Work out the finished part from the listing and answer in its coordinate system (mm). A direction names the side the tool comes from. Round coordinates to 2 decimals unless told otherwise and drop trailing zeros. Order: outer loops, then holes, each group sorted by start corner. A loop starts at its lowest first (then second) coordinate and runs counter-clockwise, first axis right, second up. Notation, with made-up numbers: (-14, 80.5) -> (-1, 80.5) arc R22 cw to (-1, 86.5) -> close; hole circle Ø10 at (53, 13.5). An arc over 180 degrees is marked (long way). Use a Markdown table: item, result. Add a question column.
Item 1: A cutting plane is placed at B-B, the plane y = -11.5. Determine the outline of the cut face in (x, z).
Item 2: A tool of negligible diameter and unlimited length cuts with its end or side. For faces 1 (the flat face through (6, 16, -0.15)), 2 (the cylindrical face through (-0.81, 18.34, -0.07)), 3 (the flat face through (0.996, 16.1, -6.2)), from which of +Z, -Z, +X, -X, +Y, -Y can it reach the whole face along a straight path? Write none if from no direction.
Item 3: A cutting plane is placed at A-A, the plane x = -13. Determine the outline of the cut face in (y, z).
Item 4: Find the intervals of material crossed by L1, parallel to Z at x = 1.2, y = 0; L2, parallel to Y at x = 2.5, z = 0; L3, parallel to X at y = -15, z = -4.5, in increasing order. Write a range as [from, to].
Item 5: A cutting plane is placed at C-C, the plane y = 8. Determine the outline of the cut face in (x, z).
Item 6: Flat-ended cylindrical pins translate along their axes: P1, Ø18, axis at y = 0, z = 0, coming from the +X side; P2, Ø3, axis at x = -3, y = 12.5, coming from the -Z side; P3, Ø3, axis at y = 17, z = 5.5, coming from the -X side; P4, Ø2.5, axis at y = 0, z = -22, coming from the +X side. Find the tip coordinate at first contact, or state that the pin passes through.
Item 7: For a pull along Y with two mould halves and no side action, classify faces 4 (the cylindrical face through (2.03, 0.07, 23.5)), 5 (the cylindrical face through (-7.643, 11.528, 0.14)), 6 (the cylindrical face through (1.97, 6.45, -17.26)), 7 (the flat face through (4, 0, -20)) as +Y half, -Y half, draft (parallel to the pull), parting line (faces both ways), or undercut.
from build123d import *

# Parameters (mm, degrees)
SKETCH_1_R          = 17
EXTRUDE_1_DEPTH     = 7
EXTRUDE_2_DEPTH     = 4
SKETCH_2_R          = 15
CUT_EXTRUDE_1_DEPTH = 3
CUT_EXTRUDE_2_REACH = 33.321
SKETCH_3_R          = 5.15
SKETCH_4_R          = 13
CUT_EXTRUDE_3_DEPTH = 2
CUT_EXTRUDE_4_REACH = 33.321
SKETCH_6_R          = 1.5
FILLET_1_R          = 10
FILLET_2_R          = 5
SKETCH_8_W          = 0.3
SKETCH_8_H          = 2.22932804
CUT_EXTRUDE_5_DEPTH = 3
SKETCH_9_W          = 20
SKETCH_9_H          = 2.594823192
EXTRUDE_3_DEPTH     = 8
SKETCH_10_W         = 5.99596414
SKETCH_10_H         = 20
EXTRUDE_4_DEPTH     = 8
SKETCH_11_W         = 20
SKETCH_11_H         = 6
EXTRUDE_5_DEPTH     = 10
SKETCH_12_R         = 3
CUT_EXTRUDE_6_DEPTH = 10
FILLET_3_R          = 10
EXTRUDE_6_DEPTH     = 3
FILLET_5_R          = 5
FILLET_6_R          = 5
FILLET_7_R          = 8
FILLET_9_R          = 2


with BuildPart() as part:
    # 草图1 → 凸台-拉伸1 (new body)
    with BuildSketch(Plane(origin=(0, 0, 0), x_dir=(0, 0, -1), z_dir=(1, 0, 0))):
        Circle(SKETCH_1_R)
    extrude(amount=EXTRUDE_1_DEPTH)

    # 草图5 → 凸台-拉伸2 (add)
    with BuildSketch(Plane.ZY):
        Polygon((0, 5.000073493), (26, 5.000073493), (26, -4.999926507), (11, -4.999926507), (-26, -4.999926507), (-26, 5.000073493), align=None)
    extrude(amount=-EXTRUDE_2_DEPTH)

    # 草图2 → 切除-拉伸1 (cut)
    with BuildSketch(Plane(origin=(7, 0, 0), x_dir=(0, 0, -1), z_dir=(1, 0, 0))):
        Circle(SKETCH_2_R)
    extrude(amount=-CUT_EXTRUDE_1_DEPTH, mode=Mode.SUBTRACT)

    # 草图3 → 切除-拉伸2 (cut, up to next)
    with BuildSketch(Plane(origin=(4, 0, 0), x_dir=(0, 0, -1), z_dir=(1, 0, 0)), mode=Mode.PRIVATE) as cut_extrude_2_sk1:
        Circle(SKETCH_3_R)
    cut_extrude_2_tool1 = extrude(cut_extrude_2_sk1.sketch, amount=-CUT_EXTRUDE_2_REACH, mode=Mode.PRIVATE) & part.part
    add(cut_extrude_2_tool1.solids().sort_by_distance((4, 0, 0))[0], mode=Mode.SUBTRACT)

    # 草图4 → 切除-拉伸3 (cut)
    with BuildSketch(Plane(origin=(4, 0, 0), x_dir=(0, 0, -1), z_dir=(1, 0, 0))):
        Circle(SKETCH_4_R)
    extrude(amount=-CUT_EXTRUDE_3_DEPTH, mode=Mode.SUBTRACT)

    # 草图6 → 切除-拉伸4 (cut, up to next)
    with BuildSketch(Plane(origin=(4, 0, 0), x_dir=(0, 0, -1), z_dir=(1, 0, 0)), mode=Mode.PRIVATE) as cut_extrude_4_sk1:
        with Locations((-22, 7.3493e-05)):
            Circle(SKETCH_6_R)
    cut_extrude_4_tool1 = extrude(cut_extrude_4_sk1.sketch, amount=-CUT_EXTRUDE_4_REACH, mode=Mode.PRIVATE) & part.part
    # 草图6 → 切除-拉伸4 (cut, up to next)
    with BuildSketch(Plane(origin=(4, 0, 0), x_dir=(0, 0, -1), z_dir=(1, 0, 0)), mode=Mode.PRIVATE) as cut_extrude_4_sk2:
        with Locations((22, 7.3493e-05)):
            Circle(SKETCH_6_R)
    cut_extrude_4_tool2 = extrude(cut_extrude_4_sk2.sketch, amount=-CUT_EXTRUDE_4_REACH, mode=Mode.PRIVATE) & part.part
    add(cut_extrude_4_tool1.solids().sort_by_distance((4, 7.3e-05, 22))[0], mode=Mode.SUBTRACT)
    add(cut_extrude_4_tool2.solids().sort_by_distance((4, 7.3e-05, -22))[0], mode=Mode.SUBTRACT)

    # 圆角1
    fillet_1_edges = [part.edges().sort_by_distance(p)[0] for p in [
        (2, 5.000073493, -16.248054193),
        (2, 5.000073493, 16.248054193),
        (2, -4.999926507, 16.248099425),
        (2, -4.999926507, -16.248099425),
    ]]
    fillet(fillet_1_edges, radius=FILLET_1_R)

    # 圆角2
    fillet_2_edges = [part.edges().sort_by_distance(p)[0] for p in [
        (2, 5.000073493, 26),
        (2, -4.999926507, 26),
        (2, -4.999926507, -26),
        (2, 5.000073493, -26),
    ]]
    fillet(fillet_2_edges, radius=FILLET_2_R)

    # 草图8 → 切除-拉伸5 (cut)
    with BuildSketch(Plane(origin=(7, 0, 0), x_dir=(0, 0, -1), z_dir=(1, 0, 0))):
        with Locations((0, 16.113914001)):
            Rectangle(SKETCH_8_W, SKETCH_8_H)
    extrude(amount=-CUT_EXTRUDE_5_DEPTH, mode=Mode.SUBTRACT)

    # 草图9 → 凸台-拉伸3 (add)
    with BuildSketch(Plane.ZY):
        with Locations((0, 12.450315489)):
            Rectangle(SKETCH_9_W, SKETCH_9_H)
    extrude(amount=EXTRUDE_3_DEPTH)

    # 草图10 → 凸台-拉伸4 (add)
    with BuildSketch(Plane(origin=(0, 13.747727085, 0), x_dir=(1, 0, 0), z_dir=(0, 1, 0))):
        with Locations((-5.00201793, 0)):
            Rectangle(SKETCH_10_W, SKETCH_10_H)
    extrude(amount=EXTRUDE_4_DEPTH)

    # 草图11 → 凸台-拉伸5 (add)
    with BuildSketch(Plane.ZY.offset(8)):
        with Locations((0, 18.747727085)):
            Rectangle(SKETCH_11_W, SKETCH_11_H)
    extrude(amount=EXTRUDE_5_DEPTH)

    # 草图12 → 切除-拉伸6 (cut)
    with BuildSketch(Plane(origin=(0, 21.747727085, 0), x_dir=(1, 0, 0), z_dir=(0, 1, 0))):
        with Locations(Location((-13, 0, 0), (0, 0, 270))):
            Circle(SKETCH_12_R)
    extrude(amount=-CUT_EXTRUDE_6_DEPTH, mode=Mode.SUBTRACT)

    # 圆角3
    # the kernel refuses this fillet: 10 mm, written as the material it adds along each edge
    with BuildSketch(Plane(origin=(0, 11.152903893, 10), x_dir=(0, -1, 0), z_dir=(0, 0, -1))) as fillet_3_piece_1_section:
        with BuildLine():
            CenterArc((9.797958971, 10), FILLET_3_R, 191.536959033, 78.463040967)
            Line((0, 8), (0, 0))
            Line((0, 0), (9.797958971, 0))
        make_face()
    fillet_3_piece_1 = extrude(amount=20, mode=Mode.PRIVATE)
    fillet_3_piece_1 = fillet_3_piece_1 - Plane(origin=(0, 0, 0), x_dir=(0, 0, -1), z_dir=(1, 0, 0)) * Cylinder(5.15, 80, mode=Mode.PRIVATE)
    add(fillet_3_piece_1)

    # 草图13 → 凸台-拉伸6 (add)
    with BuildSketch(Plane(origin=(-2.00403586, 0, 0), x_dir=(0, 0, -1), z_dir=(1, 0, 0))):
        Polygon((0, 17), (10, 17), (10, 13.747727085), (-10, 13.747727085), (-10, 17), align=None)
    extrude(amount=EXTRUDE_6_DEPTH)

    # 圆角5
    # the kernel refuses this fillet: 5 mm, written as the material it takes off along each edge
    with BuildSketch(Plane(origin=(-2.00403586, 17, -10), x_dir=(0, -1, 0), z_dir=(1, 0, 0))) as fillet_5_piece_1_section:
        with BuildLine():
            CenterArc((FILLET_5_R, -FILLET_5_R), FILLET_5_R, 90, 90)
            Line((0, -FILLET_5_R), (0, 0))
            Line((0, 0), (FILLET_5_R, 0))
        make_face()
    fillet_5_piece_1 = extrude(amount=15.5, mode=Mode.PRIVATE)
    fillet_5_piece_1 = split(fillet_5_piece_1, bisect_by=Plane(origin=(0, 17, -10), z_dir=(-1, 0, 0)), keep=Keep.TOP, mode=Mode.PRIVATE)
    add(fillet_5_piece_1, mode=Mode.SUBTRACT)
    with BuildSketch(Plane(origin=(-2.00403586, 17, -10), x_dir=(0, -1, 0), z_dir=(1, 0, 0))) as fillet_5_piece_2_section:
        with BuildLine():
            CenterArc((FILLET_5_R, -FILLET_5_R), FILLET_5_R, 90, 90)
            Line((0, -FILLET_5_R), (0, 0))
            Line((0, 0), (FILLET_5_R, 0))
        make_face()
    fillet_5_piece_2 = extrude(amount=15.5, mode=Mode.PRIVATE)
    fillet_5_piece_2 = fillet_5_piece_2 - Plane(origin=(-2.00403586, 0, 0), x_dir=(0, 0, -1), z_dir=(-1, 0, 0)) * Cylinder(17, 51, mode=Mode.PRIVATE)
    add(fillet_5_piece_2, mode=Mode.SUBTRACT)
    with BuildSketch(Plane(origin=(-2.00403586, 17, 10), x_dir=(0, -1, 0), z_dir=(1, 0, 0))) as fillet_5_piece_3_section:
        with BuildLine():
            CenterArc((FILLET_5_R, FILLET_5_R), FILLET_5_R, 180, 90)
            Line((0, FILLET_5_R), (0, 0))
            Line((0, 0), (FILLET_5_R, 0))
        make_face()
    fillet_5_piece_3 = extrude(amount=15.5, mode=Mode.PRIVATE)
    fillet_5_piece_3 = split(fillet_5_piece_3, bisect_by=Plane(origin=(0, 17, 10), z_dir=(-1, 0, 0)), keep=Keep.TOP, mode=Mode.PRIVATE)
    add(fillet_5_piece_3, mode=Mode.SUBTRACT)
    with BuildSketch(Plane(origin=(-2.00403586, 17, 10), x_dir=(0, -1, 0), z_dir=(1, 0, 0))) as fillet_5_piece_4_section:
        with BuildLine():
            CenterArc((FILLET_5_R, FILLET_5_R), FILLET_5_R, 180, 90)
            Line((0, FILLET_5_R), (0, 0))
            Line((0, 0), (FILLET_5_R, 0))
        make_face()
    fillet_5_piece_4 = extrude(amount=15.5, mode=Mode.PRIVATE)
    fillet_5_piece_4 = fillet_5_piece_4 - Plane(origin=(-2.00403586, 0, 0), x_dir=(0, 0, -1), z_dir=(-1, 0, 0)) * Cylinder(17, 51, mode=Mode.PRIVATE)
    add(fillet_5_piece_4, mode=Mode.SUBTRACT)

    # 圆角6
    # the kernel refuses this fillet: 5 mm, written as the material it adds along each edge
    with BuildSketch(Plane(origin=(-2.00403586, 12, -5), x_dir=(0, 1, 0), z_dir=(0, 0, 1))) as fillet_6_piece_1_section:
        with BuildLine():
            CenterArc((9.582575695, -5), FILLET_6_R, 90, 66.421821522)
            Line((5, -3), (5, 0))
            Line((5, 0), (9.582575695, 0))
        make_face()
    fillet_6_piece_1 = revolve(axis=Axis((-2.00403586, 12, -5), (-1, 0, 0)), revolution_arc=221.333860008, mode=Mode.PRIVATE)
    fillet_6_piece_1 = fillet_6_piece_1 - Plane(origin=(-10, 1.354944922, -5), x_dir=(0, -1, 0), z_dir=(0, 0, 1)) * Cylinder(10, 39, mode=Mode.PRIVATE)
    fillet_6_piece_1 = split(fillet_6_piece_1, bisect_by=Plane(origin=(-2.00403586, 12, -10), z_dir=(0, 0, 1)), keep=Keep.TOP, mode=Mode.PRIVATE)
    add(fillet_6_piece_1)
    with BuildSketch(Plane(origin=(-2.00403586, 12, 5), x_dir=(0, 1, 0), z_dir=(0, 0, -1))) as fillet_6_piece_2_section:
        with BuildLine():
            CenterArc((9.582575695, 5), FILLET_6_R, 203.578178478, 66.421821522)
            Line((5, 3), (5, 0))
            Line((5, 0), (9.582575695, 0))
        make_face()
    fillet_6_piece_2 = revolve(axis=Axis((-2.00403586, 12, 5), (1, 0, 0)), revolution_arc=221.333860008, mode=Mode.PRIVATE)
    fillet_6_piece_2 = fillet_6_piece_2 - Plane(origin=(-10, 1.354944922, 5), x_dir=(0, -1, 0), z_dir=(0, 0, 1)) * Cylinder(10, 39, mode=Mode.PRIVATE)
    fillet_6_piece_2 = split(fillet_6_piece_2, bisect_by=Plane(origin=(-2.00403586, 12, 10), z_dir=(0, 0, -1)), keep=Keep.TOP, mode=Mode.PRIVATE)
    add(fillet_6_piece_2)
    with BuildSketch(Plane(origin=(-2.00403586, 17, -5), x_dir=(0, 1, 0), z_dir=(0, 0, 1))) as fillet_6_piece_3:
        with BuildLine():
            CenterArc((4.582575695, -5), FILLET_6_R, 90, 66.421821522)
            Line((0, -3), (0, 0))
            Line((0, 0), (4.582575695, 0))
        make_face()
    extrude(amount=10)

    # 圆角7
    fillet_7_edges = [part.edges().sort_by_distance(p)[0] for p in [
        (-18, 18.747727085, -10),
        (-18, 18.747727085, 10),
    ]]
    fillet(fillet_7_edges, radius=FILLET_7_R)

    # 圆角9
    fillet_9_edges = [part.edges().sort_by_distance(p)[0] for p in [
        (-2.00403586, 21.747727085, 0),
        (-8, 11.152903893, 0),
    ]]
    fillet(fillet_9_edges, radius=FILLET_9_R)


solid = part.part
Reported:
| question | item | result |
|---|---|---|
| 1 | outline | (0, -12.52) -> (7, -12.52) -> (7, -9.63) -> (4, -9.63) -> (4, -6.06) -> (2, -6.06) -> (2, 6.06) -> (4, 6.06) -> (4, 9.63) -> (7, 9.63) -> (7, 12.52) -> (0, 12.52) -> close |
| 2 | face 1 | +X, +Y |
| 2 | face 2 | +Z, -Z, +X, +Y |
| 2 | face 3 | -Z, +X, +Y |
| 3 | outline | (15.75, -9.42) -> (21.75, -9.42) -> (21.75, -3) -> (15.75, -3) -> close; (15.75, 3) -> (21.75, 3) -> (21.75, 9.42) -> (15.75, 9.42) -> close |
| 4 | L1 | [-26, -23.5], [-20.5, -5.15], [5.15, 20.5], [23.5, 26] |
| 4 | L2 | [-17, -13], [13, 17] |
| 4 | L3 | [0, 7] |
| 5 | outline | (-2.53, -10) -> (0, -10) -> (0, -15.31) -> (4, -15.31) -> (4, -15) -> (7, -15) -> (7, -12.69) -> (4, -12.69) -> (4, -10.25) -> (2, -10.25) -> (2, 10.25) -> (4, 10.25) -> (4, 12.69) -> (7, 12.69) -> (7, 15) -> (4, 15) -> (4, 15.31) -> (0, 15.31) -> (0, 10) -> (-2.53, 10) -> close |
| 6 | P1 | x = 2 |
| 6 | P2 | z = -10 |
| 6 | P3 | x = -17.75 |
| 6 | P4 | through |
| 7 | face 4 | undercut |
| 7 | face 5 | -Y half |
| 7 | face 6 | +Y half |
| 7 | face 7 | draft |
